For this review, take the finished solid that the model builds, in its own axes (mm). Face numbers are marked on the shaded views. Round coordinates to 2 decimals unless told otherwise and drop trailing zeros. Write each loop counter-clockwise with the first axis right and the second up, starting at its lowest first coordinate (ties: lowest second). Pieces come first, ordered by that corner, then holes. Notation, with made-up numbers: (56, 11.25) - (105, 11.25) arc R25 cw to (105, 36.25) - close; hole circle Ø6 at (1.5, -32). An arc over 180 degrees is marked (long way). One line per item, written item: value. Start each with the question number.
Q1. Add section A-A on z = -17.5. Write out the cut boundary in (x, y), and give its area (3 significant figures).
Q2. For probe 1 along Z at (x, y) = (4, 7.25); probe 2 along X at (y, z) = (10.25, -14.75); probe 3 along X at (y, z) = (2, -11), list the stretches that pass through material, from the lowest coordinate up.
Q3. Mouldability with a two-part tool opening along Y and no side actions: class the marked faces 1, 2 and 3 as +Y half, -Y half, draft (parallel to the pull), parting line (faces both ways), or undercut.
Q4. Clearance check with flat-ended pins moving along their axes: pin 1 Ø12 at (y, z) = (9.5, -7) entering from +X; pin 2 Ø1 at (y, z) = (4, -20) entering from +X; pin 3 Ø9 at (x, y) = (-2, 6) entering from -Z; pin 4 Ø6 at (x, z) = (-14, -6) entering from -Y. State where each tip first meets the part, or that it passes through.
Q5. Add section B-B on z = -20.5. Write out the cut boundary in (x, y), and give its area (3 significant figures).
```python
from build123d import *

# Parameters (mm, degrees)
F1_ANGLE = 120
F4_R     = 2
F5_DEPTH = 10
F7_DEPTH = 25
F9_DEPTH = 19


with BuildPart() as f1:
    # F0 (on Front) → F1 (revolve)
    with BuildSketch(Plane.XZ):
        Polygon((0, -3), (0, 0), (-15, 0), (-21.162831, -23), (-13, -23), (-11, -21), (-11, -3), align=None)
    revolve(axis=Axis((0, 0, -1.5), (0, 0, -1)), revolution_arc=F1_ANGLE)

    # F4 (on face) → F5 (join)
    with BuildSketch(Plane(origin=(-0.502405, 0.870191, -3.75), x_dir=(0.991591, 0.029252, -0.12606), z_dir=(-0.12941, 0.224144, -0.965926))):
        with Locations((-7.787523, -13.964204)):
            Circle(F4_R)
    extrude(amount=F5_DEPTH)

    # F6 (on face) → F7 (cut)
    with BuildSketch(Plane.XY):
        with BuildLine():
            Line((-15, 20), (-15, 0))
            ThreePointArc((-15, 0), (-10.606602, 10.606602), (0, 15))
            Line((0, 15), (0, 20))
            Line((0, 20), (-15, 20))
        make_face()
    extrude(amount=F7_DEPTH, mode=Mode.SUBTRACT)

    # F8 (on face) → F9 (cut)
    with BuildSketch(Plane(origin=(0, 0, -23), x_dir=(1, 0, 0), z_dir=(0, 0, -1))):
        with BuildLine():
            Line((-10.452272, -1), (-11.707369, -1))
            ThreePointArc((-11.707369, -1), (-5.875, -10.175798), (4.987659, -10.638879))
            Line((4.987659, -10.638879), (4.360111, -9.551933))
            ThreePointArc((4.360111, -9.551933), (-5.25, -9.093267), (-10.452272, -1))
        make_face()
    extrude(amount=-F9_DEPTH, mode=Mode.SUBTRACT)


solid = f1.part
```
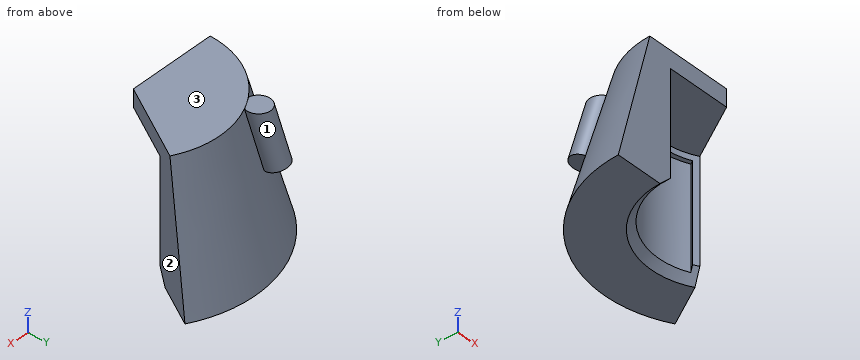
Result set:
1. outline: (-19.69, 0) - (-11, 0) arc R11 cw to (-10.95, 1) - (-11.71, 1) arc R11.75 cw to (4.99, 10.64) - (4.61, 9.99) arc R11 cw to (5.5, 9.53) - (9.84, 17.05) arc R19.69 ccw to start
1. area: 263 mm^2
2. probe 1: z = -3 to 0
2. probe 2: x = -15.94 to -5.74, 4.76 to 5.92
2. probe 3: x = -17.84 to -11.58
3. face 1: undercut
3. face 2: -Y half
3. face 3: draft
4. pin 1: stops at x = 8.72
4. pin 2: stops at x = -10.85
4. pin 3: stops at z = -3
4. pin 4: stops at y = 0
5. outline: (-20.49, 0) - (-11, 0) arc R11 cw to (-10.95, 1) - (-11.71, 1) arc R11.75 cw to (4.99, 10.64) - (4.61, 9.99) arc R11 cw to (5.5, 9.53) - (10.25, 17.75) arc R20.49 ccw to start
5. area: 297 mm^2
